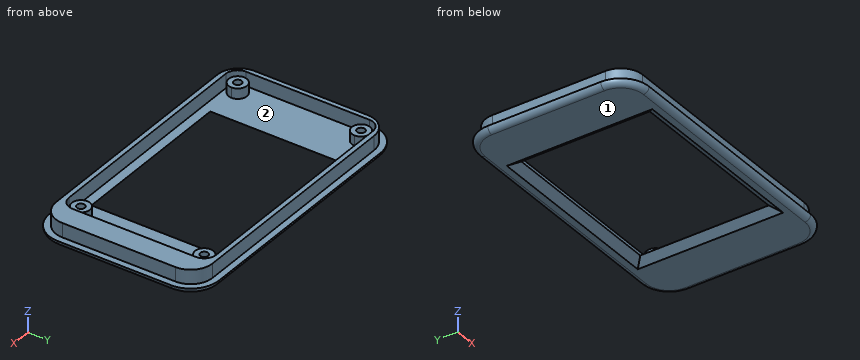
```python
from build123d import *

# Parameters (mm, degrees)
F1_DEPTH = 5.6
F2_DEPTH = 7
F0_W     = 59.6
F0_H     = 45.2
F3_DEPTH = 2
F4_R     = 1.99999
F5_SIZE2 = 1.99999
F5_SIZE  = 2.99999
F6_R     = 1.4
F7_DEPTH = 5


# Not quite as in the source:
# - a fillet or chamfer is up to 0.001 mm smaller than in the source, because OpenCascade refuses the exact size


with BuildPart() as f1:
    # F0 (on Top) → F1 (new body)
    with BuildSketch(Plane.XY):
        with BuildLine():
            ThreePointArc((-34.4414402544, 28.5581715763), (-31.2414402544, 25.3581715763), (-28.0414402544, 28.5581715763))
            ThreePointArc((-28.0414402544, 28.5581715763), (-28.9786985547, 30.8209132761), (-31.2414402544, 31.7581715763))
            ThreePointArc((-31.2414402544, 31.7581715763), (-33.5041819542, 30.8209132761), (-34.4414402544, 28.5581715763))
        make_face()
    extrude(amount=F1_DEPTH)



with BuildPart() as f1b:
    # F0 (on Top) → F1, piece 2 (new body)
    with BuildSketch(Plane.XY):
        with BuildLine():
            ThreePointArc((-28.0414402544, -14.8418284237), (-31.2414402544, -11.6418284237), (-34.4414402544, -14.8418284237))
            ThreePointArc((-34.4414402544, -14.8418284237), (-33.5041819542, -17.1045701235), (-31.2414402544, -18.0418284237))
            ThreePointArc((-31.2414402544, -18.0418284237), (-28.9786985547, -17.1045701235), (-28.0414402544, -14.8418284237))
        make_face()
    extrude(amount=F1_DEPTH)


with BuildPart() as f1c:
    # F0 (on Top) → F1, piece 3 (new body)
    with BuildSketch(Plane.XY):
        with BuildLine():
            ThreePointArc((47.3585597456, -18.0418284237), (49.6213014453, -17.1045701235), (50.5585597456, -14.8418284237))
            ThreePointArc((50.5585597456, -14.8418284237), (45.0958180458, -12.5790867239), (47.3585597456, -18.0418284237))
        make_face()
    extrude(amount=F1_DEPTH)


with BuildPart() as f1d:
    # F0 (on Top) → F1, piece 4 (new body)
    with BuildSketch(Plane.XY):
        with BuildLine():
            ThreePointArc((50.5585597456, 28.5581715763), (49.6213014453, 30.8209132761), (47.3585597456, 31.7581715763))
            ThreePointArc((47.3585597456, 31.7581715763), (45.0958180458, 26.2954298765), (50.5585597456, 28.5581715763))
        make_face()
    extrude(amount=F1_DEPTH)


with BuildPart() as f2:
    # F0 (on Top) → F2 (new body)
    with BuildSketch(Plane.XY):
        with BuildLine():
            Line((51.5585597456, 34.4581715763), (-29.4414402544, 34.4581715763))
            ThreePointArc((-29.4414402544, 34.4581715763), (-34.8861624696, 32.2028937914), (-37.1414402544, 26.7581715763))
            Line((-37.1414402544, 26.7581715763), (-37.1414402544, -13.0418284237))
            ThreePointArc((-37.1414402544, -13.0418284237), (-34.8861624696, -18.4865506389), (-29.4414402544, -20.7418284237))
            Line((-29.4414402544, -20.7418284237), (51.5585597456, -20.7418284237))
            ThreePointArc((51.5585597456, -20.7418284237), (57.0032819607, -18.4865506389), (59.2585597456, -13.0418284237))
            Line((59.2585597456, -13.0418284237), (59.2585597456, 26.7581715763))
            ThreePointArc((59.2585597456, 26.7581715763), (57.0032819607, 32.2028937914), (51.5585597456, 34.4581715763))
        make_face()
        with BuildLine():
            ThreePointArc((47.3585597456, 32.7581715763), (50.3284082265, 31.5280200572), (51.5585597456, 28.5581715763))
            Line((51.5585597456, 28.5581715763), (51.5585597456, -14.8418284237))
            ThreePointArc((51.5585597456, -14.8418284237), (50.3284082265, -17.8116769047), (47.3585597456, -19.0418284237))
            Line((47.3585597456, -19.0418284237), (-31.2414402544, -19.0418284237))
            ThreePointArc((-31.2414402544, -19.0418284237), (-34.2112887354, -17.8116769047), (-35.4414402544, -14.8418284237))
            Line((-35.4414402544, -14.8418284237), (-35.4414402544, 28.5581715763))
            ThreePointArc((-35.4414402544, 28.5581715763), (-34.2112887354, 31.5280200572), (-31.2414402544, 32.7581715763))
            Line((-31.2414402544, 32.7581715763), (47.3585597456, 32.7581715763))
        make_face(mode=Mode.SUBTRACT)
    extrude(amount=F2_DEPTH)


with BuildPart() as f1_1:
    add(f1.part)

    add(f1b.part)  # F3 merges F1b

    add(f1c.part)  # F3 merges F1c

    add(f1d.part)  # F3 merges F1d

    add(f2.part)  # F3 merges F2
    # F0 (on Top) → F3 (join)
    with BuildSketch(Plane.XY):
        with BuildLine():
            Line((51.5585597456, 36.7581715763), (-29.4414402544, 36.7581715763))
            ThreePointArc((-29.4414402544, 36.7581715763), (-36.5125080663, 33.8292393881), (-39.4414402544, 26.7581715763))
            Line((-39.4414402544, 26.7581715763), (-39.4414402544, -13.0418284237))
            ThreePointArc((-39.4414402544, -13.0418284237), (-36.5125080663, -20.1128962356), (-29.4414402544, -23.0418284237))
            Line((-29.4414402544, -23.0418284237), (51.5585597456, -23.0418284237))
            ThreePointArc((51.5585597456, -23.0418284237), (58.6296275574, -20.1128962356), (61.5585597456, -13.0418284237))
            Line((61.5585597456, -13.0418284237), (61.5585597456, 26.7581715763))
            ThreePointArc((61.5585597456, 26.7581715763), (58.6296275574, 33.8292393881), (51.5585597456, 36.7581715763))
        make_face()
        with BuildLine():
            ThreePointArc((-37.1414402544, 26.7581715763), (-34.8861624696, 32.2028937914), (-29.4414402544, 34.4581715763))
            Line((-29.4414402544, 34.4581715763), (51.5585597456, 34.4581715763))
            ThreePointArc((51.5585597456, 34.4581715763), (57.0032819607, 32.2028937914), (59.2585597456, 26.7581715763))
            Line((59.2585597456, 26.7581715763), (59.2585597456, -13.0418284237))
            ThreePointArc((59.2585597456, -13.0418284237), (57.0032819607, -18.4865506389), (51.5585597456, -20.7418284237))
            Line((51.5585597456, -20.7418284237), (-29.4414402544, -20.7418284237))
            ThreePointArc((-29.4414402544, -20.7418284237), (-34.8861624696, -18.4865506389), (-37.1414402544, -13.0418284237))
            Line((-37.1414402544, -13.0418284237), (-37.1414402544, 26.7581715763))
        make_face(mode=Mode.SUBTRACT)
        with BuildLine():
            Line((51.5585597456, -14.8418284237), (51.5585597456, 28.5581715763))
            ThreePointArc((51.5585597456, 28.5581715763), (50.3284082265, 31.5280200572), (47.3585597456, 32.7581715763))
            Line((47.3585597456, 32.7581715763), (-31.2414402544, 32.7581715763))
            ThreePointArc((-31.2414402544, 32.7581715763), (-34.2112887354, 31.5280200572), (-35.4414402544, 28.5581715763))
            Line((-35.4414402544, 28.5581715763), (-35.4414402544, -14.8418284237))
            ThreePointArc((-35.4414402544, -14.8418284237), (-34.2112887354, -17.8116769047), (-31.2414402544, -19.0418284237))
            Line((-31.2414402544, -19.0418284237), (47.3585597456, -19.0418284237))
            ThreePointArc((47.3585597456, -19.0418284237), (50.3284082265, -17.8116769047), (51.5585597456, -14.8418284237))
        make_face()
        with BuildLine():
            ThreePointArc((-34.4414402544, 28.5581715763), (-33.5041819542, 30.8209132761), (-31.2414402544, 31.7581715763))
            Line((-31.2414402544, 31.7581715763), (47.3585597456, 31.7581715763))
            ThreePointArc((47.3585597456, 31.7581715763), (49.6213014453, 30.8209132761), (50.5585597456, 28.5581715763))
            Line((50.5585597456, 28.5581715763), (50.5585597456, -14.8418284237))
            ThreePointArc((50.5585597456, -14.8418284237), (49.6213014453, -17.1045701235), (47.3585597456, -18.0418284237))
            Line((47.3585597456, -18.0418284237), (-31.2414402544, -18.0418284237))
            ThreePointArc((-31.2414402544, -18.0418284237), (-33.5041819542, -17.1045701235), (-34.4414402544, -14.8418284237))
            Line((-34.4414402544, -14.8418284237), (-34.4414402544, 28.5581715763))
        make_face(mode=Mode.SUBTRACT)
        with BuildLine():
            ThreePointArc((-31.2414402544, 31.7581715763), (-28.9786985547, 30.8209132761), (-28.0414402544, 28.5581715763))
            ThreePointArc((-28.0414402544, 28.5581715763), (-31.2414402544, 25.3581715763), (-34.4414402544, 28.5581715763))
            Line((-34.4414402544, 28.5581715763), (-34.4414402544, -14.8418284237))
            ThreePointArc((-34.4414402544, -14.8418284237), (-31.2414402544, -11.6418284237), (-28.0414402544, -14.8418284237))
            ThreePointArc((-28.0414402544, -14.8418284237), (-28.9786985547, -17.1045701235), (-31.2414402544, -18.0418284237))
            Line((-31.2414402544, -18.0418284237), (47.3585597456, -18.0418284237))
            ThreePointArc((47.3585597456, -18.0418284237), (45.0958180458, -12.5790867239), (50.5585597456, -14.8418284237))
            Line((50.5585597456, -14.8418284237), (50.5585597456, 28.5581715763))
            ThreePointArc((50.5585597456, 28.5581715763), (45.0958180458, 26.2954298765), (47.3585597456, 31.7581715763))
            Line((47.3585597456, 31.7581715763), (-31.2414402544, 31.7581715763))
        make_face()
        with Locations((11.0585597456, 6.8581715763)):
            Rectangle(F0_W, F0_H, mode=Mode.SUBTRACT)
    extrude(amount=F3_DEPTH)

    # F4 (radius 2 in the source; OpenCascade refuses exactly that, so slightly less here)
    f4_edges = [f1_1.edges().sort_by_distance(p)[0] for p in [
        (-36.512508, -20.112896, 0),
    ]]
    fillet(f4_edges, radius=F4_R)

    # F5 (size 3 and 2 in the source; OpenCascade refuses exactly that, so slightly less here)
    f5_edges = [f1_1.edges().sort_by_distance(p)[0] for p in [
        (11.05856, 29.458172, 0),
        (-18.74144, 6.858172, 0),
        (11.05856, -15.741828, 0),
        (40.85856, 6.858172, 0),
    ]]
    f5_side = f1_1.faces().sort_by_distance((-34.307016, -17.907405, 0))[0]
    chamfer(f5_edges, length=F5_SIZE, length2=F5_SIZE2, reference=f5_side)

    # F6 (on face) → F7 (cut)
    with BuildSketch(Plane.XY.offset(5.6)):
        with Locations((-31.2414402544, 28.5581715763)):
            Circle(F6_R)
        with Locations((-31.2414402544, -14.8418284237)):
            Circle(F6_R)
        with Locations((47.3585597456, -14.8418284237)):
            Circle(F6_R)
        with Locations((47.3585597456, 28.5581715763)):
            Circle(F6_R)
    extrude(amount=-F7_DEPTH, mode=Mode.SUBTRACT)


solid = f1_1.part
```
Geometry: final body of the model. Coordinates: model frame, mm. Face numbers are marked on the shaded views. Give positions to 0.01 mm unless a question says otherwise; leave off trailing zeros. Write each question's results on one line, items separated by ' | '. Start each with the question number.
1) First-contact query: pin 1 (1.5 mm diameter, centred on x = 36.5, z = 5.5, fed in from -Y); pin 2 (1.9 mm diameter, centred on x = -32.5, y = 29, fed in from +Z); pin 3 (5 mm diameter, centred on x = -1.5, y = 28, fed in from -Z); pin 4 (2 mm diameter, centred on x = 27.5, z = 1, fed in from +Y). Flat tips, straight axial feed; report the tip coordinate or a pass-through.
2) Draft query along Y for the marked faces 1 and 2. Return one class per face: pulls with the +Y half, pulls with the -Y half, needs draft (parallel to the pull), parting line crosses it, or undercut.
3) Line query: line 1 (Y direction, x = 26, z = 4); line 2 (X direction, y = 10.5, z = 4); line 3 (X direction, y = -16.5, z = 4.25). Output: solid intervals per line, ascending. Write a range as from..to.
Calculated:
1) pin 1: y = -20.74 | pin 2: z = 5.6 | pin 3: z = 1.31 | pin 4: y = 36.76
2) face 1: needs draft | face 2: undercut
3) line 1: -20.74..-19.04, 32.76..34.46 | line 2: -37.14..-35.44, 51.56..59.26 | line 3: -36.32..-35.1, -33.98..-28.5, 44.62..50.1, 51.22..58.44
